from build123d import *

# Parameters (mm, degrees)
SKETCH1_R               = 50
BOSS_EXTRUDE1_DEPTH     = 175
SKETCH4_R               = 60
BOSS_EXTRUDE3_DEPTH     = 250
BOSS_EXTRUDE4_DEPTH     = 62.5
CUT_EXTRUDE2_DEPTH      = 616.817546031
CUT_EXTRUDE2_DEPTH_BACK = 616.817546031
SKETCH6_R               = 12.5
CHAMFER2_SIZE           = 30
CHAMFER3_SIZE           = 7.5
CUT_EXTRUDE3_DEPTH      = 609.712781203
CUT_EXTRUDE3_DEPTH_BACK = 609.712781203


with BuildPart() as part:
    # Sketch1 → Boss-Extrude1 (new body)
    with BuildSketch(Plane(origin=(0, 0, 0), x_dir=(1, 0, 0), z_dir=(0, 1, 0))):
        with Locations(Location((0, 0, 0), (0, 0, 270))):
            Circle(SKETCH1_R)
    extrude(amount=BOSS_EXTRUDE1_DEPTH)

    # Sketch4 → Boss-Extrude3 (add)
    with BuildSketch(Plane(origin=(0, 175, 0), x_dir=(1, 0, 0), z_dir=(0, 1, 0))):
        with Locations(Location((0, 0, 0), (0, 0, 270))):
            Circle(SKETCH4_R)
    extrude(amount=BOSS_EXTRUDE3_DEPTH)

    # Sketch5 → Boss-Extrude4 (add, symmetric)
    with BuildSketch(Plane(origin=(0, 0, 0), x_dir=(0, 0, -1), z_dir=(1, 0, 0))):
        Polygon((-62.5, 425), (62.5, 425), (82.5, 455), (82.5, 590), (62.5, 590), (62.5, 460), (-62.5, 460), (-62.5, 590), (-82.5, 590), (-82.5, 455), align=None)
    extrude(amount=BOSS_EXTRUDE4_DEPTH, both=True)

    # Sketch6 → Cut-Extrude2 (cut, two sides: drawn at the far end of the back side and taken through both)
    with BuildSketch(Plane.XY.offset(82.5).offset(-CUT_EXTRUDE2_DEPTH_BACK)):
        with Locations(Location((0, 527.5, 0), (0, 0, 90))):
            Circle(SKETCH6_R)
        with BuildLine():
            Line((-62.5, 527.5), (-67.5, 527.5))
            Line((-67.5, 527.5), (-67.5, 595))
            Line((-67.5, 595), (67.5, 595))
            Line((67.5, 595), (67.5, 527.5))
            Line((67.5, 527.5), (62.5, 527.5))
            ThreePointArc((62.5, 527.5), (0, 590), (-62.5, 527.5))
        make_face()
    extrude(amount=CUT_EXTRUDE2_DEPTH + CUT_EXTRUDE2_DEPTH_BACK, mode=Mode.SUBTRACT)

    # Chamfer2
    # the kernel refuses this chamfer: 30 mm, written as the material it adds along each edge
    with BuildSketch(Plane(origin=(0, 425, 0), x_dir=(0, 0, 1), z_dir=(-1, 0, 0))) as chamfer2_piece_1_section:
        Polygon((60 + CHAMFER2_SIZE, 0), (60, -CHAMFER2_SIZE), (60, 0), align=None)
    chamfer2_piece_1 = revolve(axis=Axis((0, 425, 0), (0, 1, 0)), mode=Mode.PRIVATE)
    chamfer2_piece_1 = split(chamfer2_piece_1, bisect_by=Plane(origin=(-62.5, 399.085825085, 31.840161024), z_dir=(1, 0, 0)), keep=Keep.TOP, mode=Mode.PRIVATE)
    chamfer2_piece_1 = split(chamfer2_piece_1, bisect_by=Plane(origin=(54.930093835, 392.908722455, 41.10581497), z_dir=(0, 0.5547001962252294, -0.8320502943378435)), keep=Keep.TOP, mode=Mode.PRIVATE)
    chamfer2_piece_1 = split(chamfer2_piece_1, bisect_by=Plane(origin=(54.930093835, 363.517804586, -21.511869724), z_dir=(0, 0.5547001962252294, 0.8320502943378435)), keep=Keep.TOP, mode=Mode.PRIVATE)
    chamfer2_piece_1 = split(chamfer2_piece_1, bisect_by=Plane(origin=(62.5, 399.085825085, 31.840161024), z_dir=(-1, 0, 0)), keep=Keep.TOP, mode=Mode.PRIVATE)
    add(chamfer2_piece_1)

    # Chamfer3
    chamfer3_edges = [part.edges().sort_by_distance(p)[0] for p in [
        (-62.5, 438.486605007, 71.491070005),
        (-62.5, 438.486605007, -71.491070005),
        (-62.5, 491.25, -82.5),
        (62.5, 438.486605007, 71.491070005),
        (62.5, 438.486605007, -71.491070005),
        (62.5, 491.25, -82.5),
        (-62.5, 491.25, 82.5),
        (62.5, 491.25, 82.5),
        (0, 590, -82.5),
    ]]
    chamfer(chamfer3_edges, length=CHAMFER3_SIZE)

    # Sketch7 → Cut-Extrude3 (cut, two sides: drawn at the far end of the back side and taken through both)
    with BuildSketch(Plane.ZY.offset(62.5).offset(-CUT_EXTRUDE3_DEPTH_BACK)):
        with BuildLine():
            Line((-62.5, 460), (62.5, 460))
            ThreePointArc((62.5, 460), (0, 426.457809879), (-62.5, 460))
        make_face()
    extrude(amount=CUT_EXTRUDE3_DEPTH + CUT_EXTRUDE3_DEPTH_BACK, mode=Mode.SUBTRACT)


solid = part.part
Work out the finished part from the listing and answer in its coordinate system (mm). A direction names the side the tool comes from. Give positions to 0.01 mm unless a question says otherwise; leave off trailing zeros. Loops run counter-clockwise (first coordinate to the right, second up) from the corner with the lowest first, then second, coordinate; pieces in that order, holes last. Notation, with made-up numbers: (3, 38) -> (62, 38) arc R18 ccw to (62, 65) -> close; hole circle Ø9 at (14.25, -37.5). An arc over 180 degrees is marked (long way). Use a Markdown table: item, result. Add a question column.
1) The part is cut by section A-A, the plane x = 0. Determine the outline of the cut face in (y, z).
2) For a pull along Y with two mould halves and no side action, classify faces 4 (the conical face through (1.22, 582.956, 82.031)), 5 (the flat face through (1, 504, -82.5)), 6 (the conical face through (60.818, 395.822, 0.67)), 7 (the cylindrical face through (-0.55, 515.012, -72.64)) as +Y half, -Y half, draft (parallel to the pull), parting line (faces both ways), or undercut.
3) The part is cut by section D-D, the plane y = 166. Determine the outline of the cut face in (x, z).
4) Each of these flat-tipped pins is pushed along its axis until it touches: P1, Ø6, axis at x = 34.5, y = 379.5, coming from the +Z side; P2, Ø2, axis at y = 179.5, z = -50.5, coming from the +X side; P3, Ø6, axis at x = -25.5, z = -56, coming from the +Y side; P4, Ø5, axis at x = 47, z = -10, coming from the -Y side. Where does it stop, or does it pass through?
5) Which of the six approach directions +Z, -Z, +X, -X, +Y, -Y give full straight-line access (tool end or side, diameter ignored) to faces 1 (the flat face through (1, 511, -62.5)), 2 (the cylindrical face through (15.02, 86.28, 47.69)), 3 (the conical face through (-60.818, 395.822, -0.67))?
6) Consider line 1 along X through (y, z) = (527.5, 69.5); line 2 along Z through (x, y) = (-26.5, 509); line 3 along X through (y, z) = (345, -1). Determine where each line is inside the solid, lowest interval first.
7) The part is cut by section B-B, the plane z = 0. Determine the outline of the cut face in (x, y).
8) The part is cut by section C-C, the plane y = 225. Determine the outline of the cut face in (x, z), plus the area to 3 significant figures.
Reported:
| question | item | result |
|---|---|---|
| 1 | outline | (0, -50) -> (175, -50) -> (175, -60) -> (421.25, -60) -> (455, -82.5) -> (515, -82.5) -> (515, -62.5) -> (460, -62.5) arc R75 cw to (460, 62.5) -> (515, 62.5) -> (515, 82.5) -> (455, 82.5) -> (421.25, 60) -> (175, 60) -> (175, 50) -> (0, 50) -> close; (540, -82.5) -> (582.5, -82.5) -> (590, -75) -> (590, -62.5) -> (540, -62.5) -> close; (540, 62.5) -> (590, 62.5) -> (590, 75) -> (582.5, 82.5) -> (540, 82.5) -> close |
| 2 | face 4 | +Y half |
| 2 | face 5 | draft |
| 2 | face 6 | -Y half |
| 2 | face 7 | undercut |
| 3 | outline | circle Ø100 at (0, 0) |
| 4 | P1 | stops at z = 51.07 |
| 4 | P2 | stops at x = 33.91 |
| 4 | P3 | stops at y = 455.15 |
| 4 | P4 | stops at y = 0 |
| 5 | face 1 | +X, -X, +Y |
| 5 | face 2 | -Y |
| 5 | face 3 | -X, -Y |
| 6 | line 1 | x = -62.5 to -12.5, 12.5 to 62.5 |
| 6 | line 2 | z = -82.5 to -62.5, 62.5 to 82.5 |
| 6 | line 3 | x = -59.99 to 59.99 |
| 7 | outline | (-62.5, 397.5) -> (-60, 395) -> (-60, 175) -> (-50, 175) -> (-50, 0) -> (50, 0) -> (50, 175) -> (60, 175) -> (60, 395) -> (62.5, 397.5) -> (62.5, 426.46) -> (-62.5, 426.46) -> close |
| 8 | outline | circle Ø120 at (0, 0) |
| 8 | area | 11,300 mm^2 |
